```python
from build123d import *

# Parameters (mm, degrees)
SKETCH1_W           = 101.6
SKETCH1_H           = 28.215251418
SKETCH1_R           = 3.175
BOSS_EXTRUDE1_DEPTH = 3.175
CHAMFER1_SIZE       = 3.175


with BuildPart() as part:
    # Sketch1 → Boss-Extrude1 (new body)
    with BuildSketch(Plane.XY):
        with Locations((50.8, 14.107625709)):
            Rectangle(SKETCH1_W, SKETCH1_H)
        with Locations((5.2076336, 14.107625709)):
            Circle(SKETCH1_R, mode=Mode.SUBTRACT)
        with Locations((15.3676336, 14.107625709)):
            Circle(SKETCH1_R, mode=Mode.SUBTRACT)
        with Locations((25.5276336, 14.107625709)):
            Circle(SKETCH1_R, mode=Mode.SUBTRACT)
        with Locations((35.6876336, 14.107625709)):
            Circle(SKETCH1_R, mode=Mode.SUBTRACT)
        with Locations((45.8476336, 14.107625709)):
            Circle(SKETCH1_R, mode=Mode.SUBTRACT)
        with Locations((56.0076336, 14.107625709)):
            Circle(SKETCH1_R, mode=Mode.SUBTRACT)
        with Locations((66.1676336, 14.107625709)):
            Circle(SKETCH1_R, mode=Mode.SUBTRACT)
        with Locations((76.3276336, 14.107625709)):
            Circle(SKETCH1_R, mode=Mode.SUBTRACT)
        with Locations((86.4876336, 14.107625709)):
            Circle(SKETCH1_R, mode=Mode.SUBTRACT)
        with Locations((96.6476336, 14.107625709)):
            Circle(SKETCH1_R, mode=Mode.SUBTRACT)
    extrude(amount=BOSS_EXTRUDE1_DEPTH)

    # Chamfer1
    chamfer1_edges = [part.edges().sort_by_distance(p)[0] for p in [
        (50.8, 0, 3.175),
        (50.8, 28.215251418, 3.175),
    ]]
    chamfer(chamfer1_edges, length=CHAMFER1_SIZE - 0.0001)  # a hair under: the kernel refuses the full size


solid = part.part
```
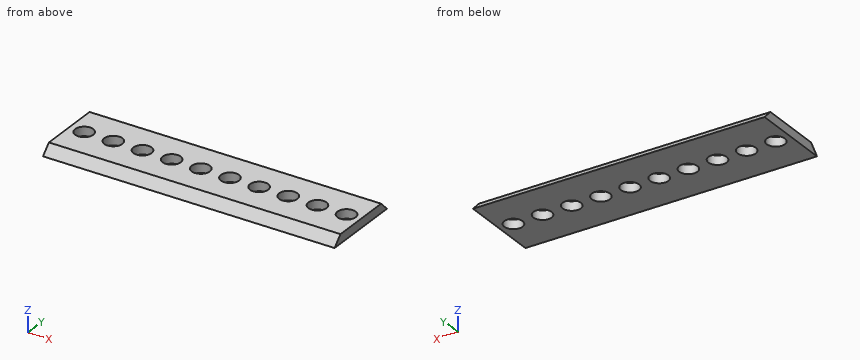
Geometry: final body of the model. Coordinates: model frame, mm. Coordinates: 2 decimals unless noted, no trailing zeros. Answer in a Markdown table with one row per item.
Item 1: Section B-B on z = 2.5. State how many separate pieces and enclosed holes the cut face has, plus the area to 3 significant figures.
Return value:
| item | result |
|---|---|
| separate pieces | 1 |
| enclosed holes | 10 |
| area | 2,040 mm² |
Item 2: Ray query, L1, parallel to Y at x = 58.5, z = 0.2; L2, parallel to Y at x = 33.5, z = 2.3; L3, parallel to Y at x = 80.5, z = 1.2. Return the intervals inside material, ascending.
Return value:
| item | result |
|---|---|
| L1 | y = 0.2 to 12.14, 16.07 to 28.02 |
| L2 | y = 2.3 to 11.81, 16.41 to 25.92 |
| L3 | y = 1.2 to 27.02 |
Item 3: Contact query for a flat-ended pin moving along its axis: P1, Ø1.5, axis at x = 79, z = 1.5, coming from the -Y side. Output: stop coordinate, or through.
Return value:
| item | result |
|---|---|
| P1 | stops at y = 0.75 |
